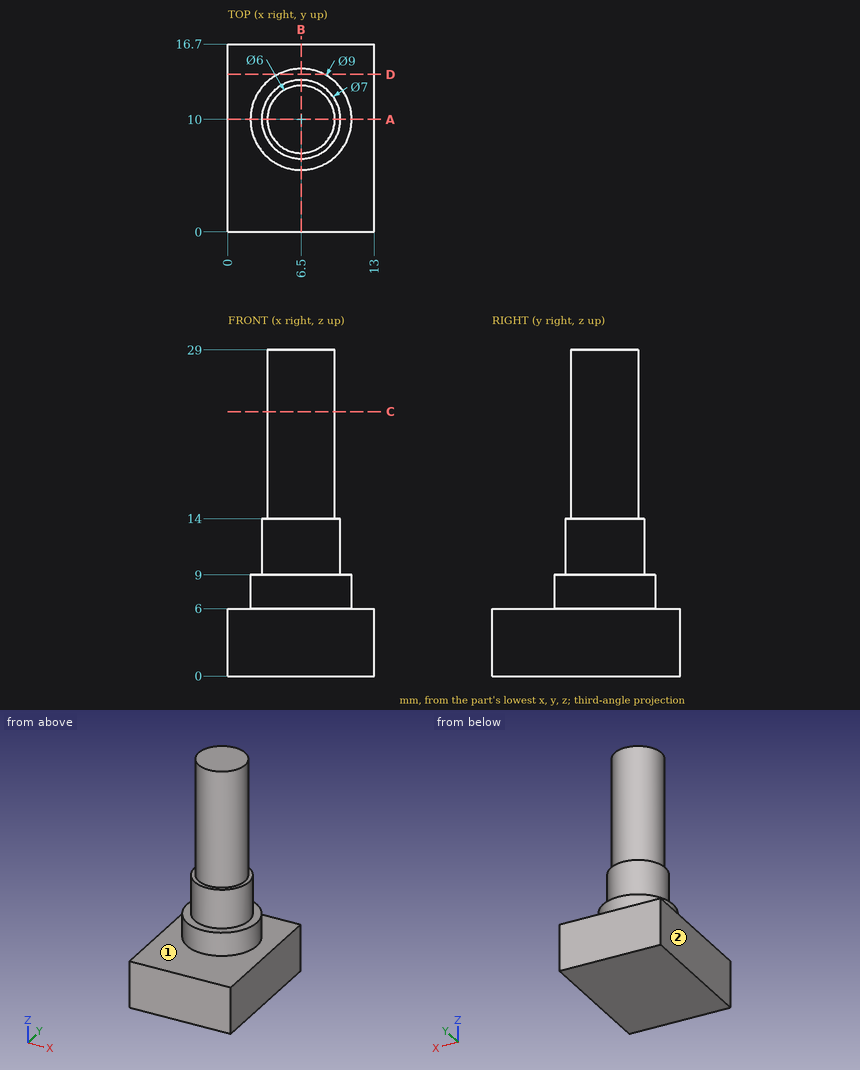
Part print with two shaded views. Sizes in mm from the minimum x, y, z corner. A direction names the side the tool comes from. Coordinates: 2 decimals unless noted, no trailing zeros. Write each loop counter-clockwise with the first axis right and the second up, starting at its lowest first coordinate (ties: lowest second). Pieces come first, ordered by that corner, then holes. Notation, with made-up numbers: (30.25, 26.5) - (41.25, 26.5) arc R14 cw to (41.25, 34.5) - close; hole circle Ø5 at (20, 61). An arc over 180 degrees is marked (long way). Use a Markdown table: item, result. Add a question column.
Item 1: Drill centre lines: line 1 along Z through (x, y) = (3.5, 5.75); line 2 along Z through (x, y) = (2.5, 11); line 3 along Y through (x, z) = (3.75, 24.25). Where is each one in solid material? Low to high.
Item 2: Band-saw the part on D-D, the plane y = 14. Write the cut outline in (x, z), and give its area (3 significant figures).
Item 3: Band-saw the part on C-C, the plane z = 23.5. Write the cut outline in (x, y).
Item 4: Band-saw the part on A-A, the plane y = 10. Write the cut outline in (x, z), and give its area (3 significant figures).
Item 5: 3-axis set-ups, long thin cutter, end or side, ignore diameter. For the marked faces 1 and 2: which of +Z, -Z, +X, -X, +Y, -Y reach the whole face in a straight line?
Item 6: Band-saw the part on B-B, the plane x = 6.5. Write the cut outline in (y, z).
Item 7: Drop flat-ended pins along their axis: pin 1 (1.5 mm diameter, centred on x = 5, z = 23.5, fed in from -Y); pin 2 (3 mm diameter, centred on y = 7, z = 19, fed in from +X); pin 3 (3 mm diameter, centred on x = 5.5, z = 23.5, fed in from +Y). Give the stop position or say it passes through.
A:
| question | item | result |
|---|---|---|
| 1 | line 1 | z = 0 to 6 |
| 1 | line 2 | z = 0 to 9 |
| 1 | line 3 | y = 8.8 to 11.2 |
| 2 | outline | (0, 0) - (13, 0) - (13, 6) - (8.56, 6) - (8.56, 9) - (4.44, 9) - (4.44, 6) - (0, 6) - close |
| 2 | area | 90.4 mm² |
| 3 | outline | circle Ø6 at (6.5, 10) |
| 4 | outline | (0, 0) - (13, 0) - (13, 6) - (11, 6) - (11, 9) - (10, 9) - (10, 14) - (9.5, 14) - (9.5, 29) - (3.5, 29) - (3.5, 14) - (3, 14) - (3, 9) - (2, 9) - (2, 6) - (0, 6) - close |
| 4 | area | 230 mm² |
| 5 | face 1 | +Z |
| 5 | face 2 | +Z, -Z, -X, +Y, -Y |
| 6 | outline | (0, 0) - (16.7, 0) - (16.7, 6) - (14.5, 6) - (14.5, 9) - (13.5, 9) - (13.5, 14) - (13, 14) - (13, 29) - (7, 29) - (7, 14) - (6.5, 14) - (6.5, 9) - (5.5, 9) - (5.5, 6) - (0, 6) - close |
| 7 | pin 1 | stops at y = 7.1 |
| 7 | pin 2 | stops at x = 9.1 |
| 7 | pin 3 | stops at y = 13 |
